Part print with two shaded views. Sizes in mm from the minimum x, y, z corner. Round coordinates to 2 decimals unless told otherwise and drop trailing zeros. Order: outer loops, then holes, each group sorted by start corner. A loop starts at its lowest first (then second) coordinate and runs counter-clockwise, first axis right, second up. Notation, with made-up numbers: M -18.5,72.25 L 1.5,72.25 A21 ccw 1.5,107.25 Z; hole C -14,35 d2. An arc over 180 degrees is marked long. Answer as a JSON object with one key per item and string values.
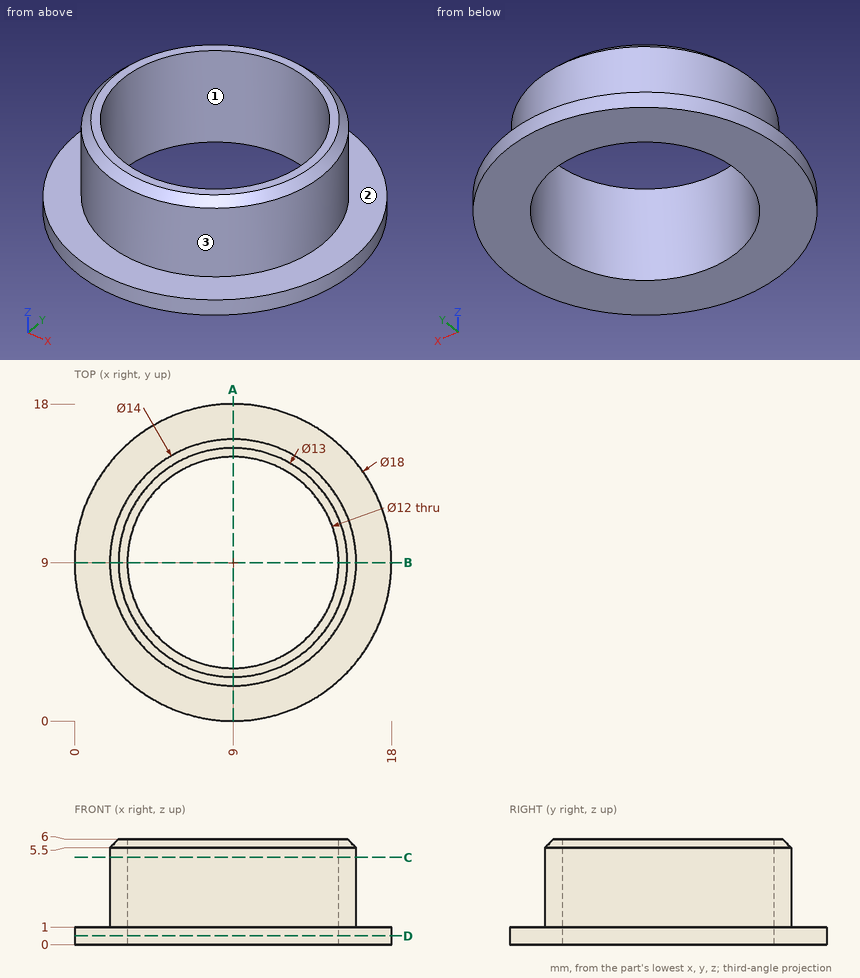
Item 1: Saw through at C-C on z = 4.95. List the corners of the cut face in (x, y), and give its area (3 significant figures).
Worked answers:
{"outline": "C 9,9 d14; hole C 9,9 d12", "area": "40.8 mm2"}
Item 2: Wall check: line 1 along Y through (x, z) = (9, 2.3); line 2 along Z through (x, y) = (8.5, 1); line 3 along X through (y, z) = (7, 4.3). Give the ranges that are in metal, low to high. Write a range as [from, to].
Worked answers:
{"line 1": "y = [2, 3], [15, 16]", "line 2": "z = [0, 1]", "line 3": "x = [2.29, 3.34], [14.66, 15.71]"}
Item 3: Two-plate mould, pull along Y, no slides. Class the marked faces 1, 2 and 3: released by +Y, released by -Y, zero draft, split by the parting line, or undercut.
Worked answers:
{"face 1": "undercut", "face 2": "zero draft", "face 3": "split by the parting line"}
Item 4: Saw through at A-A on x = 9. List the corners of the cut face in (y, z), and give its area (4 significant figures).
Worked answers:
{"outline": "M 0,0 L 3,0 L 3,6 L 2.5,6 L 2,5.5 L 2,1 L 0,1 Z; M 15,0 L 18,0 L 18,1 L 16,1 L 16,5.5 L 15.5,6 L 15,6 Z", "area": "15.75 mm2"}
Item 5: Saw through at D-D on z = 0.5. List the corners of the cut face in (x, y), and give its area (3 significant figures).
Worked answers:
{"outline": "C 9,9 d18; hole C 9,9 d12", "area": "141 mm2"}
Item 6: Drop flat-ended pins along their axis: pin 1 Ø5 at (x, y) = (9, 4.5) entering from +Z; pin 2 Ø1.5 at (x, y) = (14.5, 16) entering from +Z; pin 3 Ø1 at (y, z) = (4, 3.5) entering from -X; pin 4 Ø2 at (y, z) = (9, 2.5) entering from -X. Give the stop position or say it passes through.
Worked answers:
{"pin 1": "stops at z = 6", "pin 2": "stops at z = 1", "pin 3": "stops at x = 3.64", "pin 4": "stops at x = 2"}
